Read the model definition and answer for the solid it produces. Units are mm, in the model's axes. A direction names the side the tool comes from. Give positions to 0.01 mm unless a question says otherwise; leave off trailing zeros. Loops run counter-clockwise (first coordinate to the right, second up) from the corner with the lowest first, then second, coordinate; pieces in that order, holes last.
(1) Find section C-C, the plane z = -13. State how many separate pieces and enclosed holes the cut face has, then the cut area to 3 significant figures.
(2) Which of the six approach directions +Z, -Z, +X, -X, +Y, -Y give full straight-line access (tool end or side, diameter ignored) to faces 5 (the face through (-44.63, 16.73, 3.15)), 6 (the face through (-45.14, 0.66, 3.31)), 7 (the face through (-25.396, 7.062, -0.407))?
(3) Each of these flat-tipped pins is pushed along its axis until it touches: P1, Ø10, axis at y = 8, z = 5, coming from the +X side; P2, Ø1.5, axis at y = 15, z = -12.5, coming from the -X side; P3, Ø5, axis at x = -39, y = 10, coming from the +Z side; P4, Ø1.5, axis at x = -35, y = 7, coming from the +Z side. Where does it stop, or does it pass through?
(4) Find section D-D, the plane y = 9.5. Write down the section's boundary in (x, z), then the cut area to 3 significant figures.
(5) Determine the mould class of faces 1 (the face through (-26.66, 13.94, -7.31)), 2 (the face through (-25.4, 7.49, 0.41)), 3 (the face through (-33.43, 16.64, -9.16)), 4 (the face through (-33.39, 13.668, -9.466)) for opening direction Y: pulls with the +Y half, pulls with the -Y half, needs draft (parallel to the pull), parting line crosses it, or undercut.
(6) Find section A-A, the plane z = 0. Write down the section's boundary in (x, y).
(7) Find section B-B, the plane y = 15.25. Write down the section's boundary in (x, z).
(8) Straight lines are drawn through the part: probe 1 along X at (y, z) = (16.85, 0); probe 2 along Y at (x, z) = (-35, 14); probe 3 along Y at (x, z) = (-48, -7). For each, find the intervals that lie inside material, in ascending order.
Autodesk Inventor part; units mm, degrees
ref_plane "YZ Plane" through (0, 0, 0) normal (1, 0, 0) x (0, 1, 0)
ref_plane "XZ Plane" through (0, 0, 0) normal (0, 1, 0) x (-1, 0, 0)
ref_plane "XY Plane" through (0, 0, 0) normal (0, 0, 1) x (1, 0, 0)
sketch "Sketch1" plane through (0, 0, 0) normal (0, 0, 1) x (1, 0, 0)
  line L0 (-45.1128, 14.1503) -> (-50.5079, 10.8014)
  line L1 (-50.5079, 10.8014) -> (-45.2136, 7.2953)
  line L2 (-45.2136, 7.2953) -> (-50.6087, 3.9464)
  line L3 (-50.6087, 3.9464) -> (-45.3144, 0.4403)
  line L4 (-45.1128, 14.1503) -> (-45.1128, 19.2303)
  line L5 (-43.8697, 19.4903) -> (-45.1128, 19.2303)
  line L6 (-34.6329, 29.115) -> (-34.6329, -7.5025)
  line L7 (-43.8697, 13.8605) -> (-48.8373, 10.7769)
  line L8 (-48.8373, 10.7769) -> (-43.543, 7.2708)
  line L9 (-43.543, 7.2708) -> (-48.9149, 3.9362)
  line L10 (-43.8697, 19.4903) -> (-43.8697, 13.8605)
  line L11 (-48.9149, 3.9362) -> (-43.6359, 0.4403)
  line L12 (-43.6359, 0.4403) -> (-45.3144, 0.4403)
  point P0 (0, 0)
  dimension "d0" = 6.35
  dimension "d1" = 6.35
  dimension "d2" = 5.08
  dimension "d3" = 1.27
  dimension "d4" = 15.875
  dimension "d6" = 6.35
  dimension "d10" = 1.6784
  dimension "d11" = 19.05
revolve "Revolution1" add sketch "Sketch1" angle 360 about axis through (-34.6329, 29.115, 0) along (0, -1, 0)
properties part number "Small Suction Cup Part 1 1764"
Entries:
1. separate pieces: 2
1. enclosed holes: 2
1. area: 65.7 mm2
2. face 5: +Y
2. face 6: -Y
2. face 7: none
3. P1: stops at x = -18.78
3. P2: passes through
3. P3: stops at z = 15.75
3. P4: stops at z = 12.26
4. outline: circle Ø27.82 at (-34.63, 0); hole circle Ø24.55 at (-34.63, 0)
4. area: 134 mm2
5. face 1: pulls with the +Y half
5. face 2: undercut
5. face 3: needs draft
5. face 4: undercut
6. outline: (-50.61, 3.95) - (-45.31, 0.44) - (-43.64, 0.44) - (-48.91, 3.94) - (-43.54, 7.27) - (-48.84, 10.78) - (-43.87, 13.86) - (-43.87, 19.49) - (-45.11, 19.23) - (-45.11, 14.15) - (-50.51, 10.8) - (-45.21, 7.3) - close; (-25.72, 7.27) - (-20.35, 3.94) - (-25.63, 0.44) - (-23.95, 0.44) - (-18.66, 3.95) - (-24.05, 7.3) - (-18.76, 10.8) - (-24.15, 14.15) - (-24.15, 19.23) - (-25.4, 19.49) - (-25.4, 13.86) - (-20.43, 10.78) - close
7. outline: circle Ø20.96 at (-34.63, 0); hole circle Ø18.47 at (-34.63, 0)
8. probe 1: x = -45.11 to -43.87, -25.4 to -24.15
8. probe 2: y = 2.64 to 3.75, 4.11 to 5.17, 9.56 to 10.64, 10.9 to 11.96
8. probe 3: y = 3.36 to 4.5, 10.28 to 11.29
